Autodesk Inventor part; units mm, degrees
ref_plane "YZ Plane" through (0, 0, 0) normal (1, 0, 0) x (0, 1, 0)
ref_plane "XZ Plane" through (0, 0, 0) normal (0, 1, 0) x (-1, 0, 0)
ref_plane "XY Plane" through (0, 0, 0) normal (0, 0, 1) x (1, 0, 0)
sketch "Sketch1" plane through (0, 0, 0) normal (0, 1, 0) x (-1, 0, 0)
  line L0 (31, 0) -> (-47, 0) construction
  line L1 (0, 43) -> (0, -45) construction
  line L2 (20, 10) -> (-20, 10)
  line L3 (-20, 10) -> (-20, -10)
  line L4 (20, -10) -> (20, 10)
  line L5 (28, 12) -> (-28, 12)
  line L6 (-28, 12) -> (-28, -10)
  line L7 (28, -10) -> (28, 12)
  circle A0 centre (24.25, 5) radius 0.5
  line L8 (-20, -10) -> (-28, -10)
  line L9 (20, -10) -> (28, -10)
  circle A1 centre (24.25, -5) radius 0.5
  circle A2 centre (-24.25, 5) radius 0.5
  circle A3 centre (-24.25, -5) radius 0.5
  line L10 (-20, 10) -> (-28, 10)
  line L11 (20, 10) -> (28, 10)
  line L12 (-20, -10) -> (20, -10)
  point P0 (0, 0)
  dimension "d1" = 40
  dimension "d3" = 8
  dimension "d4" = 1
  dimension "d5" = 4.25
  dimension "d6" = 5
  dimension "d7" = 2
  dimension "d8" = 10
  dimension "d9" = 10
extrude "Extrusion1" add sketch "Sketch1" along normal blind 2 contours L11 L7 L9 L4 | L2 L10 L6 L5 L7 L11 | L3 L8 L6 L10
extrude "Extrusion2" add sketch "Sketch1" along normal blind 30 contours L2 L10 L6 L5 L7 L11
extrude "Extrusion3" add sketch "Sketch1" against normal blind 11 contours L2 L10 L6 L5 L7 L11
sketch "Sketch2" plane through (28, 0, 10) normal (0, 0, -1) x (-1, 0, 0)
  line L0 (0, 30) -> (56, 30)
  line L1 (56, 30) -> (56, 28)
  line L2 (56, -11) -> (56, 30)
  line L3 (56, 28) -> (0, 28)
  line L4 (0, 28) -> (0, 30)
  line L5 (0, 2) -> (0, 30)
  point P0 (28, 0)
  dimension "d18" = 2
extrude "Extrusion4" add sketch "Sketch2" along normal blind 20
sketch "Sketch4" plane through (-28, 30, 12) normal (0, 0, 1) x (1, 0, 0)
  line L0 (56, -41) -> (0, -41) construction
  line L1 (0, -41) -> (0, 0) construction
  line L2 (0, 0) -> (56, 0) construction
  line L3 (56, -41) -> (56, 0) construction
  line L4 (12, -46) -> (12, 10)
  line L5 (12, 10) -> (14, 10)
  line L6 (14, 10) -> (14, -46)
  line L7 (14, -46) -> (12, -46)
  line L8 (42, -46) -> (40, -46)
  line L9 (40, -46) -> (40, -38)
  line L10 (40, -38) -> (42, -38)
  line L11 (42, -38) -> (42, -46)
  line L12 (66, -18) -> (-18, -18) construction
  line L13 (42, 10) -> (40, 10)
  line L14 (40, 10) -> (40, 2)
  line L15 (40, 2) -> (42, 2)
  line L16 (42, 2) -> (42, 10)
  line L17 (42, -46) -> (12, -46)
  line L18 (12, -46) -> (12, 10)
  line L19 (12, 10) -> (42, 10)
  line L20 (42, 10) -> (42, -46)
  line L21 (0, 0) -> (2, 0)
  line L22 (2, 0) -> (2, -41)
  line L23 (2, -41) -> (0, -41)
  line L24 (0, -41) -> (0, 0)
  point P0 (28, -30)
  dimension "d32" = 2
  dimension "d33" = 12
  dimension "d35" = 56
  dimension "d36" = 2
  dimension "d37" = 8
  dimension "d38" = 3
  dimension "d39" = 28
  dimension "d52" = 2
extrude "Extrusion7" add sketch "Sketch4" along normal blind 20 contours L4 L5 L6 L7 | L9 L10 L11 L8 | L13 L16 L15 L14
extrude "Extrusion8" add sketch "Sketch4" against normal blind 2 contours L4 L5 L6 L7 | L6 L19 L14 L15 L20 L10 L9 L17 | L9 L10 L11 L8 | L13 L16 L15 L14
sketch "Sketch5" plane through (14, -11, 12) normal (1, 0, 0) x (0, 0, -1)
  line L0 (-20, -5) -> (-20, 3) construction
  line L1 (2, -5) -> (-20, -5) construction
  line L2 (-20, 3) -> (-20, 51) construction
  line L3 (-20, 51) -> (-20, 51) construction
  line L4 (-20, 51) -> (2, 51) construction
  circle A0 centre (-15, -1.25) radius 0.5
  line L5 (0, 3) -> (-20, 3) construction
  line L6 (0, -5) -> (0, 3) construction
  line L7 (-10, -8) -> (-10, 8) construction
  line L8 (8, 23) -> (-29, 23) construction
  circle A1 centre (-5, -1.25) radius 0.5
  circle A2 centre (-15, 47.25) radius 0.5
  circle A3 centre (-5, 47.25) radius 0.5
  point P0 (12, 11)
  dimension "d44" = 1
  dimension "d45" = 5
  dimension "d46" = 4.25
  dimension "d47" = 10
  dimension "d49" = 20
extrude "Extrusion9" cut sketch "Sketch5" against normal blind 6
sketch "Sketch6" plane through (0, 30, 0) normal (0, 1, 0) x (1, 0, 0)
  line L0 (28, -12) -> (-28, -12)
  line L1 (-28, -12) -> (-28, -10)
  line L2 (-28, -10) -> (28, -10)
  line L3 (28, -10) -> (28, -12)
  point P0 (0, 0)
extrude "Extrusion11" add sketch "Sketch6" along normal blind 10
sketch "Sketch7" plane through (-28, 30, 10) normal (0, 0, -1) x (-1, 0, 0)
  line L0 (0, 0) -> (0, 10)
  line L1 (-56, 10) -> (0, 10)
  line L2 (0, 10) -> (0, 8)
  line L3 (0, 8) -> (-56, 8)
  line L4 (-56, 8) -> (-56, 10)
  point P0 (-28, -30)
  dimension "d57" = 2
extrude "Extrusion12" add sketch "Sketch7" along normal blind 20
sketch "Sketch9" plane through (-28, 38, 10) normal (0, -1, 0) x (1, 0, 0)
  line L0 (56, 0) -> (56, -20) construction
  circle A0 centre (38, -10) radius 1.75
  line L1 (56, -20) -> (0, -20) construction
  line L2 (38, -13.05) -> (35.3586, -11.525)
  line L3 (35.3586, -11.525) -> (35.3586, -8.475)
  line L4 (35.3586, -8.475) -> (38, -6.95)
  line L5 (38, -6.95) -> (40.6414, -8.475)
  line L6 (40.6414, -8.475) -> (40.6414, -11.525)
  line L7 (40.6414, -11.525) -> (38, -13.05)
  line L8 (42, 0) -> (56, 0)
  line L9 (56, -20) -> (0, -20)
  line L10 (48, 0) -> (28, 0)
  line L11 (28, 0) -> (28, -20)
  line L12 (28, -20) -> (48, -20)
  line L13 (48, -20) -> (48, 0)
  line L14 (50, -10) -> (29, -10) construction
  line L15 (38, -1.4358) -> (38, -18.5642) construction
  point P0 (28, -10)
  dimension "d63" = 3.5
  dimension "d64" = 18
  dimension "d65" = 10
  dimension "d66" = 6.1
  dimension "d67" = 20
extrude "Extrusion13" add sketch "Sketch9" along normal blind 2.5 contours L8 L13 L9 L11 L10
extrude "Extrusion14" cut sketch "Sketch9" against normal blind 7.5 contours A0
properties part number "Joint"
For this review, take the finished solid that the model builds, in its own axes (mm). A direction names the side the tool comes from. Give positions to 0.01 mm unless a question says otherwise; leave off trailing zeros. Order: outer loops, then holes, each group sorted by start corner. A loop starts at its lowest first (then second) coordinate and runs counter-clockwise, first axis right, second up. Notation, with made-up numbers: M 21,82.25 L 49,82.25 A23 cw 49,91.25 Z; hole C 70.5,53.25 d5. An arc over 180 degrees is marked long. Answer in a Markdown table with one row per item. Add a question column.
(1) Consider section B-B on z = 29. State the section outline as (x, y) points, and give its area (3 significant figures).
(2) Wall thickness on probe 1 along Y at (x, z) = (13.5, 27); probe 2 along Z at (x, y) = (13.1, 36.25); probe 3 along Y at (x, z) = (-22, 7): over which ranges is each line inside the solid? List them lowest first. Write a range as [from, to].
(3) Mouldability with a two-part tool opening along Y and no side actions: class faces 6 (the face through (14, 36, 22)), 7 (the face through (11.3, 36.8, 2.3)) as +Y half, -Y half, draft (parallel to the pull), parting line (faces both ways), or undercut.
(4) Consider section C-C on x = -23. State the section outline as (y, z) points.
(5) For faces 1 (the face through (-20, 1, 0)), 2 (the face through (28, 18, 11)), 3 (the face through (20, 37, 0)), 4 (the face through (-22, 14, 12)), 5 (the face through (11.3, 36.8, -2.3)), list the 3-axis set-ups (+Z, -Z, +X, -X, +Y, -Y) from which the entire face can be reached by the end or side of a thin tool; tool diameter is ignored.
(6) For pin 1 (1 mm diameter, centred on x = 20.5, z = 11, fed in from -Y); pin 2 (4 mm diameter, centred on x = 9, z = 1.5, fed in from -Y); pin 3 (24 mm diameter, centred on y = 21.5, z = 16, fed in from -X); pin 4 (6 mm diameter, centred on y = 8.5, z = 22, fed in from +X), all flat-tipped, find the tip position at first contact; note any pin that passes through.
(7) Consider section A-A on z = 0. State the section outline as (x, y) points, and give its area (3 significant figures).
(8) Consider section D-D on y = 31. State the section outline as (x, z) points, and give its area (3 significant figures).
Evaluation:
| question | item | result |
|---|---|---|
| 1 | outline | M -16,-16 L -14,-16 L -14,40 L -16,40 Z; M 12,-16 L 14,-16 L 14,-8 L 12,-8 Z; M 12,32 L 14,32 L 14,40 L 12,40 Z |
| 1 | area | 144 mm^2 |
| 2 | probe 1 | y = [-16, -12.75], [-11.75, -8], [32, 35.75], [36.75, 40] |
| 2 | probe 2 | z = [-10, 16.5], [17.5, 26.5], [27.5, 32] |
| 2 | probe 3 | y = [0, 2], [28, 30], [38, 40] |
| 3 | face 6 | draft |
| 3 | face 7 | undercut |
| 4 | outline | M -11,10 L 0,10 L 0,-10 L 2,-10 L 2,10 L 28,10 L 28,-10 L 30,-10 L 30,10 L 38,10 L 38,-10 L 40,-10 L 40,12 L -11,12 Z |
| 5 | face 1 | -Z, -Y |
| 5 | face 2 | +Z, -Z, +X, +Y, -Y |
| 5 | face 3 | -Z, +X |
| 5 | face 4 | +Z, -X, +Y, -Y |
| 5 | face 5 | none |
| 6 | pin 1 | stops at y = -11 |
| 6 | pin 2 | stops at y = 28 |
| 6 | pin 3 | stops at x = -28 |
| 6 | pin 4 | stops at x = -14 |
| 7 | outline | M -28,0 L -20,0 L -20,2 L -28,2 Z; M -28,28 L 28,28 L 28,30 L -28,30 Z; M -28,38 L 0,38 L 0,35.5 L 7.36,35.5 L 7.36,38 L 8.25,38 L 8.25,40 L -28,40 Z; M 11.75,38 L 12.64,38 L 12.64,35.5 L 20,35.5 L 20,38 L 28,38 L 28,40 L 11.75,40 Z; M 20,0 L 28,0 L 28,2 L 20,2 Z |
| 7 | area | 286 mm^2 |
| 8 | outline | M -28,10 L 28,10 L 28,12 L -14,12 L -14,32 L -16,32 L -16,12 L -28,12 Z |
| 8 | area | 152 mm^2 |
